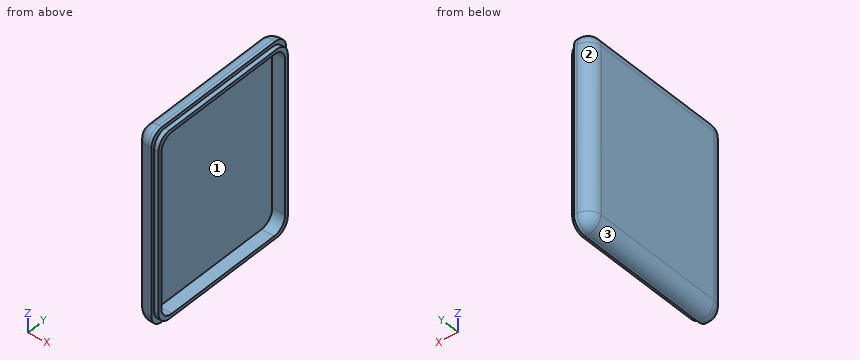
```python
from build123d import *

# Parameters (mm, degrees)
SKETCH5_W           = 76.2
SKETCH5_H           = 63.5
BOSS_EXTRUDE2_DEPTH = 6.35
SKETCH6_W           = 73.66
SKETCH6_H           = 60.96
BOSS_EXTRUDE3_DEPTH = 1.778
SKETCH7_W           = 71.12
SKETCH7_H           = 58.42
CUT_EXTRUDE2_DEPTH  = 5.08
FILLET7_R           = 5.08
FILLET8_R           = 5.08
FILLET9_R           = 5.08
FILLET10_R          = 5.08
FILLET11_R          = 5.08
FILLET12_R          = 5.08
FILLET13_R          = 5.08


with BuildPart() as part:
    # Sketch5 → Boss-Extrude2 (new body)
    with BuildSketch(Plane(origin=(0, 0, 0), x_dir=(0, 0, -1), z_dir=(1, 0, 0))):
        with Locations((65.870666667, 31.75)):
            Rectangle(SKETCH5_W, SKETCH5_H)
    extrude(amount=BOSS_EXTRUDE2_DEPTH)

    # Sketch6 → Boss-Extrude3 (add)
    with BuildSketch(Plane(origin=(6.35, 0, 0), x_dir=(0, 0, -1), z_dir=(1, 0, 0))):
        with Locations((65.870666667, 31.75)):
            Rectangle(SKETCH6_W, SKETCH6_H)
    extrude(amount=BOSS_EXTRUDE3_DEPTH)

    # Sketch7 → Cut-Extrude2 (cut)
    with BuildSketch(Plane(origin=(8.128, 0, 0), x_dir=(0, 0, -1), z_dir=(1, 0, 0))):
        with Locations((65.870666667, 31.75)):
            Rectangle(SKETCH7_W, SKETCH7_H)
    extrude(amount=-CUT_EXTRUDE2_DEPTH, mode=Mode.SUBTRACT)

    # Fillet7
    fillet7_edges = [part.edges().sort_by_distance(p)[0] for p in [
        (5.588, 2.54, -30.310666667),
        (5.588, 2.54, -101.430666667),
    ]]
    fillet(fillet7_edges, radius=FILLET7_R)

    # Fillet8
    fillet8_edges = [part.edges().sort_by_distance(p)[0] for p in [
        (5.588, 60.96, -30.310666667),
        (5.588, 60.96, -101.430666667),
    ]]
    fillet(fillet8_edges, radius=FILLET8_R)

    # Fillet9
    fillet9_edges = [part.edges().sort_by_distance(p)[0] for p in [
        (7.239, 1.27, -29.040666667),
    ]]
    fillet(fillet9_edges, radius=FILLET9_R)

    # Fillet10
    fillet10_edges = [part.edges().sort_by_distance(p)[0] for p in [
        (3.175, 0, -27.770666667),
    ]]
    fillet(fillet10_edges, radius=FILLET10_R)

    # Fillet11
    fillet11_edges = [part.edges().sort_by_distance(p)[0] for p in [
        (7.239, 1.27, -102.700666667),
        (7.239, 62.23, -102.700666667),
        (3.175, 63.5, -103.970666667),
        (3.175, 0, -103.970666667),
    ]]
    fillet(fillet11_edges, radius=FILLET11_R)

    # Fillet12
    fillet12_edges = [part.edges().sort_by_distance(p)[0] for p in [
        (7.239, 62.23, -29.040666667),
        (3.175, 63.5, -27.770666667),
    ]]
    fillet(fillet12_edges, radius=FILLET12_R)

    # Fillet13
    fillet13_edges = [part.edges().sort_by_distance(p)[0] for p in [
        (0, 31.75, -27.770666667),
        (0, 62.012102448, -29.258564218),
        (0, 0, -65.870666667),
        (0, 1.487897552, -29.258564218),
        (0, 63.5, -65.870666667),
        (0, 31.75, -103.970666667),
        (0, 1.487897552, -102.482769115),
        (0, 62.012102448, -102.482769115),
    ]]
    fillet(fillet13_edges, radius=FILLET13_R)


solid = part.part
```
Here's how the part is built. I have some questions about the finished solid (model axes, mm). Face numbers are marked on the shaded views. Round coordinates to 2 decimals unless told otherwise and drop trailing zeros. Write each loop counter-clockwise with the first axis right and the second up, starting at its lowest first coordinate (ties: lowest second). Pieces come first, ordered by that corner, then holes.
Q1. If we section it at A-A on y = 41.5: Write out the boundary of the cut face in (x, z).
Q2. If we mould it in two halves opening along Z, with no side actions, what happens to the marked faces 1, 2 and 3? For each: +Z half, -Z half, draft (parallel to the pull), parting line (faces both ways), or undercut.
Q3. Will these pins go through, and if not, where does the flat tip stop? P1, Ø2, axis at y = 18.5, z = -75.5, coming from the +X side; P2, Ø0.9, axis at x = 7, y = 40, coming from the +Z side; P3, Ø3, axis at x = 2, z = -53.5, coming from the +Y side.
Q4. If we section it at B-B on z = -93.5: Write out the boundary of the cut face in (x, y), plus the area to 3 significant figures.
Q5. Please list where these lines run through material, in increasing order: probe 1 along Y at (x, z) = (5.5, -75); probe 2 along Z at (x, y) = (6.5, 50.5); probe 3 along Z at (x, y) = (5.5, 20).
Answer below:
1. outline: (0, -98.89) arc R5.08 ccw to (5.08, -103.97) - (6.35, -103.97) - (6.35, -102.7) - (8.13, -102.7) - (8.13, -101.43) - (3.05, -101.43) - (3.05, -30.31) - (8.13, -30.31) - (8.13, -29.04) - (6.35, -29.04) - (6.35, -27.77) - (5.08, -27.77) arc R5.08 ccw to (0, -32.85) - close
2. face 1: undercut
2. face 2: draft
2. face 3: -Z half
3. P1: stops at x = 3.05
3. P2: stops at z = -29.04
3. P3: stops at y = 63.25
4. outline: (0, 5.08) arc R5.08 ccw to (5.08, 0) - (6.35, 0) - (6.35, 1.27) - (8.13, 1.27) - (8.13, 2.54) - (3.05, 2.54) - (3.05, 60.96) - (8.13, 60.96) - (8.13, 62.23) - (6.35, 62.23) - (6.35, 63.5) - (5.08, 63.5) arc R5.08 ccw to (0, 58.42) - close
4. area: 204 mm2
5. probe 1: y = 0 to 2.54, 60.96 to 63.5
5. probe 2: z = -102.7 to -101.43, -30.31 to -29.04
5. probe 3: z = -103.97 to -101.43, -30.31 to -27.77
